Build history of the part. All positions in model axes, mm. Face numbers are marked on the shaded views. Round coordinates to 2 decimals unless told otherwise and drop trailing zeros. Order: outer loops, then holes, each group sorted by start corner. A loop starts at its lowest first (then second) coordinate and runs counter-clockwise, first axis right, second up. Notation, with made-up numbers: (-33, 88.5) -> (-4, 88.5) arc R33 cw to (-4, 127.5) -> close; hole circle Ø10 at (43.25, 18.25). An arc over 180 degrees is marked (long way). Write item = value, one per line.
from build123d import *

# Parameters (mm, degrees)
REVOLVE_1_ANGLE     = 10
FILLET_1_R          = 1.5
FILLET_2_R          = 1.5
FILLET_3_R          = 1
FILLET_4_R          = 1
SKETCH_7_W          = 4
SKETCH_7_H          = 2
CUT_REVOLVE_1_ANGLE = 0.6
SKETCH_10_R         = 0.4
CUT_EXTRUDE_1_DEPTH = 2
REVOLVE_2_ANGLE     = 0.6


with BuildPart() as part:
    # 草图4 → 旋转1 (revolve)
    with BuildSketch(Plane.XY):
        Polygon((0.75, -1.5), (1.25, -1.5), (1.25, 0), (0, 0), (-1.25, 0), (-1.25, -1.5), (-0.75, -1.5), (-0.75, -4), (-2, -4), (-2, -8), (0, -8), (2, -8), (2, -4), (0.75, -4), align=None)
        Polygon((31.5, 0), (32.75, 0), (32.75, -1.5), (32.25, -1.5), (32.25, -4), (33.5, -4), (33.5, -8), (31.5, -8), (29.5, -8), (29.5, -4), (30.75, -4), (30.75, -1.5), (30.25, -1.5), (30.25, 0), align=None)
    revolve(axis=Axis((165.75, 3.853460973, 0), (0, -1, 0)), revolution_arc=REVOLVE_1_ANGLE)

    # 圆角1
    # the kernel refuses this fillet: 1.5 mm, written as the material it adds along each edge
    with BuildSketch(Plane(origin=(165.75, -4, 0), x_dir=(-1, 0, 0), z_dir=(0, 0, 1))) as fillet_1_piece_1:
        with BuildLine():
            CenterArc((163.5, -1.479019946), FILLET_1_R, 0, 80.405931773)
            Line((165, -1.479019946), (165.03, -1.479019946))
            Line((165.03, -1.479019946), (165.03, 0))
            Line((165.03, 0), (165, 0.03))
            ThreePointArc((165, 0.03), (164.375, 0.03), (163.755, 0.029580399))
            Line((163.755, 0.029580399), (163.75, 0))
        make_face()
    revolve(axis=Axis((165.75, -4, 0), (0, -1, 0)), revolution_arc=10)
    with BuildSketch(Plane(origin=(165.75, -4, 0), x_dir=(-1, 0, 0), z_dir=(0, 0, 1))) as fillet_1_piece_2:
        with BuildLine():
            CenterArc((168, -1.479019946), FILLET_1_R, 99.594068227, 80.405931773)
            Line((166.5, -1.479019946), (166.47, -1.479019946))
            Line((166.47, -1.479019946), (166.47, 0))
            Line((166.47, 0), (166.5, 0.03))
            ThreePointArc((166.5, 0.03), (167.125, 0.03), (167.745, 0.029580399))
            Line((167.745, 0.029580399), (167.75, 0))
        make_face()
    revolve(axis=Axis((165.75, -4, 0), (0, -1, 0)), revolution_arc=10)

    # 圆角2
    # the kernel refuses this fillet: 1.5 mm, written as the material it adds along each edge
    with BuildSketch(Plane(origin=(165.75, -4, 0), x_dir=(-1, 0, 0), z_dir=(0, 0, 1))) as fillet_2_piece_1:
        with BuildLine():
            CenterArc((136.5, -1.479019946), FILLET_2_R, 99.594068227, 80.405931773)
            Line((136.25, 0), (136.245, 0.029580399))
            ThreePointArc((136.245, 0.029580399), (135.625, 0.03), (135, 0.03))
            Line((135, 0.03), (134.97, 0))
            Line((134.97, 0), (134.97, -1.479019946))
            Line((134.97, -1.479019946), (135, -1.479019946))
        make_face()
    revolve(axis=Axis((165.75, -4, 0), (0, -1, 0)), revolution_arc=10)
    with BuildSketch(Plane(origin=(165.75, -4, 0), x_dir=(-1, 0, 0), z_dir=(0, 0, 1))) as fillet_2_piece_2:
        with BuildLine():
            CenterArc((132, -1.479019946), FILLET_2_R, 0, 80.405931773)
            Line((133.5, -1.479019946), (133.53, -1.479019946))
            Line((133.53, -1.479019946), (133.53, 0))
            Line((133.53, 0), (133.5, 0.03))
            ThreePointArc((133.5, 0.03), (132.875, 0.03), (132.255, 0.029580399))
            Line((132.255, 0.029580399), (132.25, 0))
        make_face()
    revolve(axis=Axis((165.75, -4, 0), (0, -1, 0)), revolution_arc=10)

    # 圆角3
    # the kernel refuses this fillet: 1 mm, written as the material it adds along each edge
    with BuildSketch(Plane(origin=(165.75, -1.5, 0), x_dir=(-1, 0, 0), z_dir=(0, 0, 1))) as fillet_3_piece_1:
        with BuildLine():
            CenterArc((136, 0.866025404), FILLET_3_R, 180, 60)
            Line((135, 0.866025404), (135, 0))
            Line((135, 0), (135.5, 0))
        make_face()
    revolve(axis=Axis((165.75, -1.5, 0), (0, -1, 0)), revolution_arc=10)
    with BuildSketch(Plane(origin=(165.75, -1.5, 0), x_dir=(-1, 0, 0), z_dir=(0, 0, 1))) as fillet_3_piece_2:
        with BuildLine():
            CenterArc((132.5, 0.866025404), FILLET_3_R, 300, 60)
            Line((133, 0), (133.5, 0))
            Line((133.5, 0), (133.5, 0.866025404))
        make_face()
    revolve(axis=Axis((165.75, -1.5, 0), (0, -1, 0)), revolution_arc=10)
    # the kernel refuses this fillet: 1 mm, written as the material it takes off along each edge
    with BuildSketch(Plane(origin=(165.75, 0, 0), x_dir=(-0.9998233399867428, 0, 0.018795978765534377), z_dir=(0.018795978765534377, 0, 0.9998233399867428))) as fillet_3_2_piece_1:
        with BuildLine():
            CenterArc((133 + FILLET_3_R, FILLET_3_R), FILLET_3_R, 180, 90)
            Line((133, FILLET_3_R), (133, 0))
            Line((133, 0), (133 + FILLET_3_R, 0))
        make_face()
    revolve(axis=Axis((165.75, 0, 0), (0, -1, 0)), revolution_arc=12.153987353, mode=Mode.SUBTRACT)
    with BuildSketch(Plane(origin=(165.75, 0, 0), x_dir=(-0.9998297984864879, 0, 0.01844922921070363), z_dir=(0.01844922921070363, 0, 0.9998297984864879))) as fillet_3_2_piece_2:
        with BuildLine():
            CenterArc((135.5 - FILLET_3_R, FILLET_3_R), FILLET_3_R, 270, 90)
            Line((135.5 - FILLET_3_R, 0), (135.5, 0))
            Line((135.5, 0), (135.5, FILLET_3_R))
        make_face()
    revolve(axis=Axis((165.75, 0, 0), (0, -1, 0)), revolution_arc=12.114245889, mode=Mode.SUBTRACT)

    # 圆角4
    # the kernel refuses this fillet: 1 mm, written as the material it adds along each edge
    with BuildSketch(Plane(origin=(165.75, -1.5, 0), x_dir=(-1, 0, 0), z_dir=(0, 0, 1))) as fillet_4_piece_1:
        with BuildLine():
            CenterArc((167.5, 0.866025404), FILLET_4_R, 180, 60)
            Line((167, 0), (166.5, 0))
            Line((166.5, 0), (166.5, 0.866025404))
        make_face()
    revolve(axis=Axis((165.75, -1.5, 0), (0, -1, 0)), revolution_arc=10)
    with BuildSketch(Plane(origin=(165.75, -1.5, 0), x_dir=(-1, 0, 0), z_dir=(0, 0, 1))) as fillet_4_piece_2:
        with BuildLine():
            CenterArc((164, 0.866025404), FILLET_4_R, 300, 60)
            Line((164.5, 0), (165, 0))
            Line((165, 0), (165, 0.866025404))
        make_face()
    revolve(axis=Axis((165.75, -1.5, 0), (0, -1, 0)), revolution_arc=10)
    # the kernel refuses this fillet: 1 mm, written as the material it takes off along each edge
    with BuildSketch(Plane(origin=(165.75, 0, 0), x_dir=(-0.9998845180351503, 0, 0.015197058715919934), z_dir=(0.015197058715919934, 0, 0.9998845180351503))) as fillet_4_2_piece_1:
        with BuildLine():
            CenterArc((164.5 + FILLET_4_R, FILLET_4_R), FILLET_4_R, 180, 90)
            Line((164.5, FILLET_4_R), (164.5, 0))
            Line((164.5, 0), (164.5 + FILLET_4_R, 0))
        make_face()
    revolve(axis=Axis((165.75, 0, 0), (0, -1, 0)), revolution_arc=11.74152169, mode=Mode.SUBTRACT)
    with BuildSketch(Plane(origin=(165.75, 0, 0), x_dir=(-0.9998879496351009, 0, 0.014969574961036002), z_dir=(0.014969574961036002, 0, 0.9998879496351009))) as fillet_4_2_piece_2:
        with BuildLine():
            CenterArc((167 - FILLET_4_R, FILLET_4_R), FILLET_4_R, 270, 90)
            Line((167 - FILLET_4_R, 0), (167, 0))
            Line((167, 0), (167, FILLET_4_R))
        make_face()
    revolve(axis=Axis((165.75, 0, 0), (0, -1, 0)), revolution_arc=11.715451006, mode=Mode.SUBTRACT)

    # 草图7 → 切除-旋转1 (revolve, cut)
    with BuildSketch(Plane.XY):
        with Locations((0, -7)):
            Rectangle(SKETCH_7_W, SKETCH_7_H)
        with Locations((31.5, -7)):
            Rectangle(SKETCH_7_W, SKETCH_7_H)
    revolve(axis=Axis((165.75, 3.853460973, 0), (0, -1, 0)), revolution_arc=CUT_REVOLVE_1_ANGLE, mode=Mode.SUBTRACT)

    # 草图10 → 切除-拉伸1 (cut)
    with BuildSketch(Plane.XZ.offset(6)):
        with Locations(Location((0.00227206, -0.867861005, 0), (0, 0, 270))):
            Circle(SKETCH_10_R)
        with Locations(Location((31.501840266, -0.702928144, 0), (0, 0, 270))):
            Circle(SKETCH_10_R)
    extrude(amount=-CUT_EXTRUDE_1_DEPTH, mode=Mode.SUBTRACT)

    # 草图11 → 旋转2 (revolve)
    with BuildSketch(Plane(origin=(4.997974052, 0, -28.344919378), x_dir=(-0.9848077530122081, 0, -0.17364817766693072), z_dir=(0.17364817766693072, 0, -0.9848077530122081))):
        Polygon((-26.981885062, -4.5), (-26.481885062, -4.5), (-22.481885062, -6), (-3.981885062, -6), (0.018114938, -4.5), (0.518114938, -4.5), (4.518114938, -4.5), (5.018114938, -4.5), (9.018114938, -6), (9.018114938, -8), (4.518114938, -8), (0.518114938, -8), (-26.981885062, -8), (-30.981885062, -8), (-35.481885062, -8), (-35.481885062, -6), (-31.481885062, -4.5), (-30.981885062, -4.5), align=None)
    revolve(axis=Axis((165.75, 3.853460973, 0), (0, 1, 0)), revolution_arc=REVOLVE_2_ANGLE)


solid = part.part
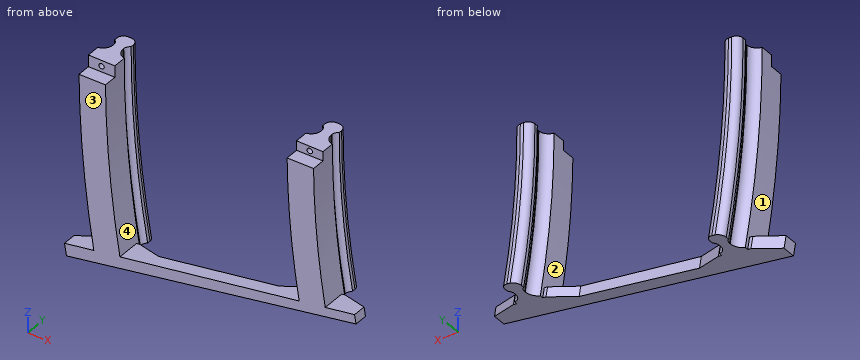
Q1. Flat gauge pins, fed straight in: pin 1 (1.4 mm diameter, centred on x = 15.5, z = -24.5, fed in from +Y); pin 2 (0.6 mm diameter, centred on x = 4.5, z = -27.5, fed in from +Y); pin 3 (0.6 mm diameter, centred on x = 0, z = -0.5, fed in from -Y); pin 4 (4 mm diameter, centred on x = 5, z = -5.5, fed in from -Y). Where does each tip first touch, or does it go through?
Check values:
pin_1 = -6
pin_2 = -3.97
pin_3 = -6
pin_4 = through
Q2. Mould opens along X. For the marked faces 1, 2, 3 and 4 say: released by +X, released by -X, zero draft, split by the parting line, or undercut.
Check values:
face_1 = released by -X
face_2 = undercut
face_3 = zero draft
face_4 = undercut
Q3. Cut at A-A, the plane y = -5. List the corners of the cut face in (x, z), and give its area (3 significant figures).
Check values:
outline = (-2, 0) arc R167.75 ccw to (0.25, -27.4) -> (-1.56, -27.7) arc R169.58 ccw to (-1.26, -29.45) -> (6.29, -28.12) arc R161.92 cw to (6.01, -26.45) -> (4.2, -26.74) arc R163.75 cw to (2, 0) -> close; (29.5, 0) arc R136.25 ccw to (31.33, -22.25) -> (29.52, -22.55) arc R138.08 ccw to (29.76, -23.98) -> (37.31, -22.65) arc R130.42 cw to (37.08, -21.3) -> (35.28, -21.6) arc R132.25 cw to (33.5, 0) -> close; hole circle Ø0.8 at (0, -0.87); hole circle Ø0.8 at (31.5, -0.7)
area = 220 mm²
Q4. Cut at C-C, the plane x = 22.5. List the corners of the cut face in (y, z), and give its area (3 significant figures).
Check values:
outline = (-8, -25.26) -> (-6, -25.26) -> (-6, -23.71) -> (-8, -23.71) -> close
area = 3.09 mm²
Q5. Cut at D-D, the plane x = 12.5. List the corners of the cut face in (y, z).
Check values:
outline = (-8, -27.02) -> (-6, -27.02) -> (-6, -25.37) -> (-8, -25.37) -> close
Q6. Cut at B-B, the plane y = -7. List the corners of the cut face in (x, z), and give its area (3 significant figures).
Check values:
outline = (-4.19, -28.13) arc R172.25 ccw to (-3.88, -29.91) -> (39.94, -22.18) arc R127.75 cw to (39.72, -20.86) -> (35.28, -21.6) arc R132.25 cw to (33.51, -1.38) -> (29.51, -1.43) arc R136.25 ccw to (31.33, -22.25) -> (4.2, -26.74) arc R163.75 cw to (2.01, -1.71) -> (-1.99, -1.76) arc R167.75 ccw to (0.25, -27.4) -> close
area = 254 mm²
Q7. Probe probe 1 along X at (y, z) = (-5.5, -5); probe 2 along X at (y, z) = (-7.25, -10); probe 3 along Z at (x, y) = (8, -6.75). List the from-to ranges inside material, lowest first.
Check values:
probe_1 = -1.93 to 2.08, 29.59 to 33.59
probe_2 = -1.7 to 2.31, 29.87 to 33.88
probe_3 = -27.82 to -26.12
